Build history of the part. All positions in model axes, mm. A direction names the side the tool comes from. Give positions to 0.01 mm unless a question says otherwise; leave off trailing zeros. Loops run counter-clockwise (first coordinate to the right, second up) from the corner with the lowest first, then second, coordinate; pieces in that order, holes last. Notation, with made-up numbers: (-11.5, -18) -> (30.5, -18) arc R11 cw to (30.5, -14) -> close; hole circle Ø6 at (-29.5, 51). An arc over 180 degrees is marked (long way). Answer as a JSON object with one key per item and string values. Group by question number.
from build123d import *

# Parameters (mm, degrees)
ESQUISSE1_W             = 116.597430489
ESQUISSE1_H             = 54.924972195
BOSS_EXTRU_1_DEPTH      = 10
CONG_1_R                = 2
COQUE2_START            = -86.741708543
COQUE2_OUTLINE_W        = 6
COQUE2_OUTLINE_H        = 50.924972195
COQUE2_DEPTH            = 112.597430489
ESQUISSE2_W             = 112.597430489
ESQUISSE2_H             = 50.924972195
ENL_V_MAT_EXTRU_2_DEPTH = 2
SUPPORT_VIS_R           = 5
SUPPORT_VIS_R_2         = 1
EX_SUPPORT_DEPTH        = 5
PAROIS_W                = 114.597430489
PAROIS_H                = 52.924972195
PAROIS_W_2              = 112.597430489
PAROIS_H_2              = 50.924972195
EX_PAROIS_DEPTH         = 5


# Read off the part's stored shape, not the designer's step: Coque2
with BuildPart() as part:
    # Esquisse1 → Boss.-Extru.1 (new body)
    with BuildSketch(Plane(origin=(0, 0, 0), x_dir=(1, 0, 0), z_dir=(0, 1, 0))):
        with Locations((-30.442993298, -10.699035797)):
            Rectangle(ESQUISSE1_W, ESQUISSE1_H)
    extrude(amount=BOSS_EXTRU_1_DEPTH)

    # Congé1
    cong_1_edges = [part.edges().sort_by_distance(p)[0] for p in [
        (-30.442993298, 0, -16.7634503),
        (27.855721946, 0, 10.699035797),
        (-30.442993298, 0, 38.161521895),
        (-88.741708543, 0, 10.699035797),
    ]]
    fillet(cong_1_edges, radius=CONG_1_R)

    # Coque2 outline → Coque2 (cut)
    with BuildSketch(Plane.YZ.offset(COQUE2_START)):
        with Locations((5, 10.699035797)):
            Rectangle(COQUE2_OUTLINE_W, COQUE2_OUTLINE_H)
    extrude(amount=COQUE2_DEPTH, mode=Mode.SUBTRACT)

    # Esquisse2 → Enlèv. mat.-Extru.2 (cut)
    with BuildSketch(Plane(origin=(0, 10, 0), x_dir=(1, 0, 0), z_dir=(0, 1, 0))):
        with Locations((-30.442993298, -10.699035797)):
            Rectangle(ESQUISSE2_W, ESQUISSE2_H)
    extrude(amount=-ENL_V_MAT_EXTRU_2_DEPTH, mode=Mode.SUBTRACT)

    # support_vis → ex_support (add)
    # profile 1 of 4: a face of its own
    with BuildSketch(Plane(origin=(0, 2, 0), x_dir=(1, 0, 0), z_dir=(0, 1, 0))):
        with Locations(Location((-80.641833666, 9.143982461, 0), (0, 0, 270))):
            Circle(SUPPORT_VIS_R)
        with Locations(Location((-80.641833666, 9.143982461, 0), (0, 0, 270))):
            Circle(SUPPORT_VIS_R_2, mode=Mode.SUBTRACT)
    # profile 2 of 4: a face of its own
    with BuildSketch(Plane(origin=(0, 2, 0), x_dir=(1, 0, 0), z_dir=(0, 1, 0))):
        with Locations(Location((20.198166334, 9.143982461, 0), (0, 0, 270))):
            Circle(SUPPORT_VIS_R)
        with Locations(Location((20.198166334, 9.143982461, 0), (0, 0, 270))):
            Circle(SUPPORT_VIS_R_2, mode=Mode.SUBTRACT)
    # profile 3 of 4: a face of its own
    with BuildSketch(Plane(origin=(0, 2, 0), x_dir=(1, 0, 0), z_dir=(0, 1, 0))):
        with Locations(Location((-80.641833666, -30.226017539, 0), (0, 0, 270))):
            Circle(SUPPORT_VIS_R)
        with Locations(Location((-80.641833666, -30.226017539, 0), (0, 0, 270))):
            Circle(SUPPORT_VIS_R_2, mode=Mode.SUBTRACT)
    # profile 4 of 4: a face of its own
    with BuildSketch(Plane(origin=(0, 2, 0), x_dir=(1, 0, 0), z_dir=(0, 1, 0))):
        with Locations(Location((20.198166334, -30.226017539, 0), (0, 0, 270))):
            Circle(SUPPORT_VIS_R)
        with Locations(Location((20.198166334, -30.226017539, 0), (0, 0, 270))):
            Circle(SUPPORT_VIS_R_2, mode=Mode.SUBTRACT)
    extrude(amount=EX_SUPPORT_DEPTH)

    # parois → ex_parois (add)
    with BuildSketch(Plane(origin=(0, 10, 0), x_dir=(1, 0, 0), z_dir=(0, 1, 0))):
        with Locations((-30.442993298, -10.699035797)):
            Rectangle(PAROIS_W, PAROIS_H)
        with Locations((-30.442993298, -10.699035797)):
            Rectangle(PAROIS_W_2, PAROIS_H_2, mode=Mode.SUBTRACT)
    extrude(amount=EX_PAROIS_DEPTH)


solid = part.part
(1) Saw through at A-A on y = 12.25. List the corners of the cut face in (x, z).
(2) Probe line 1 along X through (y, z) = (8.25, -8.5); line 2 along X through (y, z) = (11, 22); line 3 along Z through (x, y) = (-37, 4.5). List the from-to ranges inside material, lowest first. Write a range as [from, to].
(3) Pull direction Z, two halves, no side cores. Call faces 1 (the cylindrical face through (-29.63, 0.6, -16.19)), 2 (the flat face through (19, 7, -9)), 3 (the cylindrical face through (-29.63, 0.6, 37.59)): pulls with the +Z half, pulls with the -Z half, needs draft (parallel to the pull), parting line crosses it, or undercut.
(4) Saw through at D-D on z = 33. List the corners of the cut face in (x, y).
(5) 3-axis set-ups, long thin cutter, end or side, ignore diameter. For faces 4 (the cylindrical face through (-76.4, 4.5, -6.5)), 5 (the flat face through (-31, 15, -15)), 6 (the flat face through (-31, 12, -15.763)): which of +Z, -Z, +X, -X, +Y, -Y reach the whole face in a straight line?
(6) Pin check, flat tips, straight feed: pin 1 (2 mm diameter, centred on x = 20.5, z = -9, fed in from +Y); pin 2 (1 mm diameter, centred on x = 20, z = 30, fed in from +Y); pin 3 (1.5 mm diameter, centred on x = -58, y = 12, fed in from +Z). Stop position of each tip, or through.
(7) Saw through at C-C on y = 5.5. Give the number of separate pieces and of enclosed holes in the cut face, plus the area to 3 significant figures.
(8) Saw through at B-B on x = -64. List the corners of the cut face in (y, z), plus the area to 3 significant figures.
Calculated:
{
 "1": {"outline": "(-87.74, -15.76) -> (26.86, -15.76) -> (26.86, 37.16) -> (-87.74, 37.16) -> close; hole (-86.74, -14.76) -> (25.86, -14.76) -> (25.86, 36.16) -> (-86.74, 36.16) -> close"},
 "2": {"line 1": "x = [-88.74, -86.74], [25.86, 27.86]", "line 2": "x = [-87.74, -86.74], [25.86, 26.86]", "line 3": "z = [-16.76, -14.76], [36.16, 38.16]"},
 "3": {"face 1": "pulls with the -Z half", "face 2": "undercut", "face 3": "pulls with the +Z half"},
 "4": {"outline": "(-88.74, 2) arc R2 ccw to (-86.74, 0) -> (25.86, 0) arc R2 ccw to (27.86, 2) -> (27.86, 10) -> (26.86, 10) -> (26.86, 15) -> (25.86, 15) -> (25.86, 2) -> (24.36, 2) -> (24.36, 7) -> (16.04, 7) -> (16.04, 2) -> (-76.48, 2) -> (-76.48, 7) -> (-84.8, 7) -> (-84.8, 2) -> (-86.74, 2) -> (-86.74, 15) -> (-87.74, 15) -> (-87.74, 10) -> (-88.74, 10) -> close"},
 "5": {"face 4": "+Y", "face 5": "+Z, -Z, +X, -X, +Y", "face 6": "-Z, +X, -X, +Y"},
 "6": {"pin 1": "stops at y = 7", "pin 2": "stops at y = 2", "pin 3": "stops at z = 37.16"},
 "7": {"separate pieces": "5", "enclosed holes": "5", "area": "972 mm^2"},
 "8": {"outline": "(0, -14.76) arc R2 ccw to (2, -16.76) -> (10, -16.76) -> (10, -15.76) -> (15, -15.76) -> (15, -14.76) -> (2, -14.76) -> (2, 36.16) -> (15, 36.16) -> (15, 37.16) -> (10, 37.16) -> (10, 38.16) -> (2, 38.16) arc R2 ccw to (0, 36.16) -> close", "area": "150 mm^2"}
}
